The model under review builds one solid part; all positions refer to its coordinate system, in mm. A direction names the side the tool comes from. Give positions to 0.01 mm unless a question says otherwise; leave off trailing zeros. Order: outer loops, then holes, each group sorted by start corner. A loop starts at its lowest first (then second) coordinate and runs counter-clockwise, first axis right, second up. Notation, with made-up numbers: (-29.5, 5.25) -> (4.5, 5.25) arc R15 ccw to (4.5, 15.25) -> close; hole circle Ø8 at (6.5, 64.5). An arc over 180 degrees is marked (long way). Use one line per item in the form item = value.
```python
from build123d import *

# Parameters (mm, degrees)
SKETCH1_R           = 11
BOSS_EXTRUDE1_DEPTH = 7
CUT_EXTRUDE1_DEPTH  = 8
BOSS_EXTRUDE2_DEPTH = 7
BOSS_EXTRUDE3_DEPTH = 17.5
BOSS_EXTRUDE4_DEPTH = 17.5
SKETCH10_W          = 52.24
SKETCH10_H          = 17.5
CUT_EXTRUDE2_DEPTH  = 173.994845224


with BuildPart() as part:
    # Sketch1 → Boss-Extrude1 (new body)
    with BuildSketch(Plane.XY):
        with BuildLine():
            Line((42.143593539, 104.994845224), (-13.856406461, 8))
            ThreePointArc((-13.856406461, 8), (-13.856406461, -8), (0, -16))
            Line((0, -16), (112, -16))
            ThreePointArc((112, -16), (125.856406461, -8), (125.856406461, 8))
            Line((125.856406461, 8), (69.856406461, 104.994845224))
            ThreePointArc((69.856406461, 104.994845224), (56, 112.994845224), (42.143593539, 104.994845224))
        make_face()
        Circle(SKETCH1_R, mode=Mode.SUBTRACT)
        with Locations((112, 0)):
            Circle(SKETCH1_R, mode=Mode.SUBTRACT)
        with Locations((56, 96.994845224)):
            Circle(SKETCH1_R, mode=Mode.SUBTRACT)
    extrude(amount=BOSS_EXTRUDE1_DEPTH)

    # Sketch2 → Cut-Extrude1 (cut, through all)
    with BuildSketch(Plane.XY.offset(7)):
        with BuildLine():
            Line((9.622063078, 18.665902125), (23.383974596, 42.502232084))
            Line((23.383974596, 42.502232084), (48.5, 28.001488056))
            Line((48.5, 28.001488056), (48.5, -1))
            Line((48.5, -1), (20.976176963, -1))
            ThreePointArc((20.976176963, -1), (18.186533479, 10.5), (9.622063078, 18.665902125))
        make_face()
        with BuildLine():
            Line((63.5, -1), (91.023823037, -1))
            ThreePointArc((91.023823037, -1), (93.813466521, 10.5), (102.377936922, 18.665902125))
            Line((102.377936922, 18.665902125), (88.616025404, 42.502232084))
            Line((88.616025404, 42.502232084), (63.5, 28.001488056))
            Line((63.5, 28.001488056), (63.5, -1))
        make_face()
        with BuildLine():
            Line((30.883974596, 55.49261314), (44.645886115, 79.328943099))
            ThreePointArc((44.645886115, 79.328943099), (56, 75.994845224), (67.354113885, 79.328943099))
            Line((67.354113885, 79.328943099), (81.116025404, 55.49261314))
            Line((81.116025404, 55.49261314), (56, 40.991869112))
            Line((56, 40.991869112), (30.883974596, 55.49261314))
        make_face()
    extrude(amount=-CUT_EXTRUDE1_DEPTH, mode=Mode.SUBTRACT)

    # Sketch7 → Boss-Extrude2 (add)
    with BuildSketch(Plane.XY):
        with BuildLine():
            Line((-14, 156.994845224), (126, 156.994845224))
            Line((126, 156.994845224), (97.856406461, 56.497422612))
            Line((97.856406461, 56.497422612), (69.856406461, 104.994845224))
            ThreePointArc((69.856406461, 104.994845224), (56, 112.994845224), (42.143593539, 104.994845224))
            Line((42.143593539, 104.994845224), (14.143593539, 56.497422612))
            Line((14.143593539, 56.497422612), (-14, 156.994845224))
        make_face()
    extrude(amount=BOSS_EXTRUDE2_DEPTH)

    # Sketch8 → Boss-Extrude3 (add)
    with BuildSketch(Plane.XY.offset(7)):
        Polygon((-12.039699431, 149.994845224), (124.039699431, 149.994845224), (126, 156.994845224), (-14, 156.994845224), align=None)
    extrude(amount=BOSS_EXTRUDE3_DEPTH)

    # Sketch9 → Boss-Extrude4 (add)
    with BuildSketch(Plane(origin=(0, 0, 0), x_dir=(-1, 0, 0), z_dir=(0, 0, -1))):
        Polygon((-124.039699431, 149.994845224), (12.039699431, 149.994845224), (14, 156.994845224), (-126, 156.994845224), align=None)
    extrude(amount=BOSS_EXTRUDE4_DEPTH)

    # Sketch10 → Cut-Extrude2 (cut, through all)
    with BuildSketch(Plane(origin=(0, 156.994845224, 0), x_dir=(1, 0, 0), z_dir=(0, 1, 0))):
        with Locations((56, -15.75)):
            Rectangle(SKETCH10_W, SKETCH10_H)
        with Locations((56, 8.75)):
            Rectangle(SKETCH10_W, SKETCH10_H)
    extrude(amount=-CUT_EXTRUDE2_DEPTH, mode=Mode.SUBTRACT)


solid = part.part
```
1. Tool access review of faces 5 (the face through (29.88, 154, 16)), 6 (the face through (55, -16, 3)), 7 (the face through (9, 149.995, 16)), 8 (the face through (82.12, 154, -9)), 9 (the face through (16.41, 30.42, 3.55)): name each direction out of +Z, -Z, +X, -X, +Y, -Y from which nothing blocks a thin tool from reaching the whole face with its end or side.
Values:
face_5 = +Z, +Y, -Y
face_6 = +Z, -Z, +X, -X, -Y
face_7 = +Z, +X, -X, -Y
face_8 = -Z, +Y, -Y
face_9 = +Z, -Z
2. Add section C-C on y = 90.5. Give the boundary of the cut face in (x, z).
Values:
outline = (4.62, 0) -> (47.12, 0) -> (47.12, 7) -> (4.62, 7) -> close; (64.88, 0) -> (107.38, 0) -> (107.38, 7) -> (64.88, 7) -> close
3. Add section D-D on x = 115. Give the boundary of the cut face in (y, z), then the cut area to 3 significant figures.
Values:
outline = (-15.72, 0) -> (-10.58, 0) -> (-10.58, 7) -> (-15.72, 7) -> close; (10.58, 0) -> (26.8, 0) -> (26.8, 7) -> (10.58, 7) -> close; (117.72, 0) -> (149.99, 0) -> (149.99, -17.5) -> (156.99, -17.5) -> (156.99, 24.5) -> (149.99, 24.5) -> (149.99, 7) -> (117.72, 7) -> close
area = 669 mm^2
4. The part is to be moulded in two halves that separate along X. For faces 1 (the face through (35.77, 35.35, 3.55)), 2 (the face through (43.62, 48.14, 3.55)), 3 (the face through (104, 154, 24.5)), 4 (the face through (-13.97, -7.8, 3.45)), say which applies: +X half, -X half, draft (parallel to the pull), parting line (faces both ways), or undercut.
Values:
face_1 = undercut
face_2 = undercut
face_3 = draft
face_4 = -X half
5. Add section A-A on z = 12. Give the boundary of the cut face in (x, y).
Values:
outline = (-14, 156.99) -> (-12.04, 149.99) -> (29.88, 149.99) -> (29.88, 156.99) -> close; (82.12, 149.99) -> (124.04, 149.99) -> (126, 156.99) -> (82.12, 156.99) -> close
6. For L1, parallel to Y at x = 56, z = 1; L2, parallel to Z at x = 102, y = 122; L3, parallel to Y at x = 21, z = -2, list the stretches that pass through material, from the lowest coordinate up.
Values:
L1 = -16 to 40.99, 75.99 to 85.99, 107.99 to 156.99
L2 = 0 to 7
L3 = 149.99 to 156.99
7. For pin 1 Ø5 at (x, y) = (57.5, 21.5) entering from -Z; pin 2 Ø9 at (x, z) = (16, -6) entering from -Y; pin 3 Ø2 at (y, z) = (13.5, 3.5) entering from -X; pin 4 Ø10 at (x, y) = (70.5, 8.5) entering from -Z, all flat-tipped, find the tip position at first contact; note any pin that passes through.
Values:
pin_1 = 0
pin_2 = 149.99
pin_3 = -11.26
pin_4 = through
8. Add section B-B on x = 85. Give the boundary of the cut face in (y, z), then the cut area to 3 significant figures.
Values:
outline = (-16, 0) -> (-1, 0) -> (-1, 7) -> (-16, 7) -> close; (40.41, 0) -> (149.99, 0) -> (149.99, -17.5) -> (156.99, -17.5) -> (156.99, 24.5) -> (149.99, 24.5) -> (149.99, 7) -> (40.41, 7) -> close
area = 1,170 mm^2
